from build123d import *

# Parameters (mm, degrees)
CHAMFER1_SIZE                   = 2
BOSS_EXTRUDE1_DEPTH             = 70
CHAMFER3_SIZE                   = 14
SKETCH7_R                       = 5
CUT_EXTRUDE1_DEPTH              = 70
CIRPATTERN4_COUNT               = 4
CHAMFER3_OF_CIRPATTERN4_SIZE    = 14
CUT_EXTRUDE3_START              = 70
CUT_EXTRUDE3_DEPTH              = 70
CUT_EXTRUDE4_DEPTH              = 70
CIRPATTERN5_COUNT               = 2
CIRPATTERN5_ANGLE               = 10
CIRPATTERN5_THE_OTHER_WAY_COUNT = 2
CIRPATTERN5_THE_OTHER_WAY_ANGLE = 10
CIRPATTERN7_COUNT               = 4
CIRPATTERN7_COPY_1_DEPTH        = 70
CIRPATTERN7_COPY_2_DEPTH        = 70
CIRPATTERN7_COPY_3_DEPTH        = 70
CIRPATTERN7_COPY_4_DEPTH        = 70
CIRPATTERN7_COPY_5_DEPTH        = 70
CIRPATTERN7_COPY_6_DEPTH        = 70
CUT_SWEEP2_PROFILE_R            = 0.5
CUT_SWEEP9_PROFILE_R            = 0.5
CUT_EXTRUDE5_START              = -10
SKETCH109_R                     = 37.5
CUT_EXTRUDE5_DEPTH              = 10


with BuildPart() as part:
    # Sketch1 → Revolve1 (revolve)
    with BuildSketch(Plane.XY, mode=Mode.PRIVATE) as revolve1_sk:
        Polygon((0, 0), (-50, 0), (-50, 28), (-37.5, 28), (-37.5, 31), (-5, 31), (-5, 41), (0, 41), align=None)
    revolve(revolve1_sk.sketch.rotate(Axis((0, 0, 0), (0, 1, 0)), 270), axis=Axis((0, 0, 0), (0, 1, 0)))

    # Chamfer1
    chamfer1_edges = [part.edges().sort_by_distance(p)[0] for p in [
        (0, 31, 37.5),
        (0, 28, 50),
    ]]
    chamfer(chamfer1_edges, length=CHAMFER1_SIZE)

    # Sketch3 → Boss-Extrude1 (add)
    with BuildSketch(Plane.XY):
        Polygon((-12.5, 26), (-12.5, 0), (12.5, 0), (12.5, 26), (10.5, 26), (10.5, 2), (-10.5, 2), (-10.5, 26), align=None)
    boss_extrude1 = extrude(amount=BOSS_EXTRUDE1_DEPTH)

    # Chamfer3
    chamfer3_edges = [part.edges().sort_by_distance(p)[0] for p in [
        (11.5, 26, 70),
        (-11.5, 26, 70),
    ]]
    chamfer(chamfer3_edges, length=CHAMFER3_SIZE)

    # Sketch7 → Cut-Extrude1 (cut)
    with BuildSketch(Plane(origin=(0, 0, 0), x_dir=(1, 0, 0), z_dir=(0, 1, 0))):
        with Locations(Location((0, -60, 0), (0, 0, 90))):
            Circle(SKETCH7_R)
    cut_extrude1 = extrude(amount=CUT_EXTRUDE1_DEPTH, mode=Mode.SUBTRACT)

    # CirPattern4: Boss-Extrude1, Cut-Extrude1 ×4 about axis
    cirpattern4_axis = Axis((0, 0, 0), (0, 1, 0))
    add([boss_extrude1.rotate(cirpattern4_axis, i * 360 / CIRPATTERN4_COUNT) for i in range(1, CIRPATTERN4_COUNT)])
    add([cut_extrude1.rotate(cirpattern4_axis, i * 360 / CIRPATTERN4_COUNT) for i in range(1, CIRPATTERN4_COUNT)], mode=Mode.SUBTRACT)

    # Chamfer3 of CirPattern4
    chamfer3_of_cirpattern4_edges = [part.edges().sort_by_distance(p)[0] for p in [
        (70, 26, -11.5),
        (70, 26, 11.5),
        (-11.5, 26, -70),
        (11.5, 26, -70),
        (-70, 26, 11.5),
        (-70, 26, -11.5),
    ]]
    chamfer(chamfer3_of_cirpattern4_edges, length=CHAMFER3_OF_CIRPATTERN4_SIZE)

    # Sketch12 → Cut-Extrude3 (cut)
    with BuildSketch(Plane(origin=(0, 0, 0), x_dir=(1, 0, 0), z_dir=(0, 1, 0)).offset(CUT_EXTRUDE3_START)):
        with BuildLine():
            Line((23.02513458, -42.117017672), (23.12024219, -44.333445626))
            ThreePointArc((23.12024219, -44.333445626), (35.355339059, -35.355339059), (44.333445626, -23.12024219))
            Line((44.333445626, -23.12024219), (42.117017672, -23.02513458))
            ThreePointArc((42.117017672, -23.02513458), (33.941125497, -33.941125497), (23.02513458, -42.117017672))
        make_face()
    cut_extrude3 = extrude(amount=-CUT_EXTRUDE3_DEPTH, mode=Mode.SUBTRACT)

    # Sketch19 → Cut-Extrude4 (cut)
    with BuildSketch(Plane(origin=(0, 0, 0), x_dir=(1, 0, 0), z_dir=(0, 1, 0))):
        Polygon((36.062317099, -33.941125497), (33.917754876, -36.038946478), (31.819933895, -33.894384255), (33.964496118, -31.796563274), align=None)
    cut_extrude4 = extrude(amount=CUT_EXTRUDE4_DEPTH, mode=Mode.SUBTRACT)

    # CirPattern5: Cut-Extrude4 ×2 about axis
    cirpattern5_axis = Axis((0, 0, 0), (0, -1, 0))
    for i in range(1, CIRPATTERN5_COUNT):
        add(cut_extrude4.rotate(cirpattern5_axis, i * CIRPATTERN5_ANGLE / (CIRPATTERN5_COUNT - 1)), mode=Mode.SUBTRACT)

    # CirPattern5 the other way: Cut-Extrude4 ×2 about axis
    cirpattern5_the_other_way_axis = Axis((0, 0, 0), (0, 1, 0))
    for i in range(1, CIRPATTERN5_THE_OTHER_WAY_COUNT):
        add(cut_extrude4.rotate(cirpattern5_the_other_way_axis, i * CIRPATTERN5_THE_OTHER_WAY_ANGLE / (CIRPATTERN5_THE_OTHER_WAY_COUNT - 1)), mode=Mode.SUBTRACT)

    # CirPattern7: Cut-Extrude3, Cut-Extrude4 ×4 about axis
    cirpattern7_axis = Axis((0, 0, 0), (0, 1, 0))
    add([cut_extrude3.rotate(cirpattern7_axis, i * 360 / CIRPATTERN7_COUNT) for i in range(1, CIRPATTERN7_COUNT)], mode=Mode.SUBTRACT)
    add([cut_extrude4.rotate(cirpattern7_axis, i * 360 / CIRPATTERN7_COUNT) for i in range(1, CIRPATTERN7_COUNT)], mode=Mode.SUBTRACT)

    # CirPattern7 copy 1 sketch → CirPattern7 copy 1 (cut)
    with BuildSketch(Plane(origin=(0, 0, 0), x_dir=(0.1736481776669308, 0, -0.984807753012208), z_dir=(0, 1, 0))):
        Polygon((36.062317099, -33.941125497), (33.917754876, -36.038946478), (31.819933895, -33.894384255), (33.964496118, -31.796563274), align=None)
    extrude(amount=CIRPATTERN7_COPY_1_DEPTH, mode=Mode.SUBTRACT)

    # CirPattern7 copy 2 sketch → CirPattern7 copy 2 (cut)
    with BuildSketch(Plane(origin=(0, 0, 0), x_dir=(-0.984807753012208, 0, -0.17364817766693086), z_dir=(0, 1, 0))):
        Polygon((36.062317099, -33.941125497), (33.917754876, -36.038946478), (31.819933895, -33.894384255), (33.964496118, -31.796563274), align=None)
    extrude(amount=CIRPATTERN7_COPY_2_DEPTH, mode=Mode.SUBTRACT)

    # CirPattern7 copy 3 sketch → CirPattern7 copy 3 (cut)
    with BuildSketch(Plane(origin=(0, 0, 0), x_dir=(-0.17364817766693094, 0, 0.984807753012208), z_dir=(0, 1, 0))):
        Polygon((36.062317099, -33.941125497), (33.917754876, -36.038946478), (31.819933895, -33.894384255), (33.964496118, -31.796563274), align=None)
    extrude(amount=CIRPATTERN7_COPY_3_DEPTH, mode=Mode.SUBTRACT)

    # CirPattern7 copy 4 sketch → CirPattern7 copy 4 (cut)
    with BuildSketch(Plane(origin=(0, 0, 0), x_dir=(-0.1736481776669307, 0, -0.984807753012208), z_dir=(0, 1, 0))):
        Polygon((36.062317099, -33.941125497), (33.917754876, -36.038946478), (31.819933895, -33.894384255), (33.964496118, -31.796563274), align=None)
    extrude(amount=CIRPATTERN7_COPY_4_DEPTH, mode=Mode.SUBTRACT)

    # CirPattern7 copy 5 sketch → CirPattern7 copy 5 (cut)
    with BuildSketch(Plane(origin=(0, 0, 0), x_dir=(-0.984807753012208, 0, 0.17364817766693064), z_dir=(0, 1, 0))):
        Polygon((36.062317099, -33.941125497), (33.917754876, -36.038946478), (31.819933895, -33.894384255), (33.964496118, -31.796563274), align=None)
    extrude(amount=CIRPATTERN7_COPY_5_DEPTH, mode=Mode.SUBTRACT)

    # CirPattern7 copy 6 sketch → CirPattern7 copy 6 (cut)
    with BuildSketch(Plane(origin=(0, 0, 0), x_dir=(0.17364817766693055, 0, 0.984807753012208), z_dir=(0, 1, 0))):
        Polygon((36.062317099, -33.941125497), (33.917754876, -36.038946478), (31.819933895, -33.894384255), (33.964496118, -31.796563274), align=None)
    extrude(amount=CIRPATTERN7_COPY_6_DEPTH, mode=Mode.SUBTRACT)

    # Cut-Sweep2: sweep along a path in Sketch27
    with BuildLine(Plane(origin=(0, 28, 0), x_dir=(1, 0, 0), z_dir=(0, 1, 0))) as cut_sweep2_path:
        CenterArc((0, 0), 41, 0, 360)
    # Cut-Sweep2 profile (on start of the path) → Cut-Sweep2 (sweep, cut)
    with BuildSketch(Plane(origin=(41, 28, 0), x_dir=(-1, 0, 0), z_dir=(0, 0, -1))):
        Circle(CUT_SWEEP2_PROFILE_R)
    sweep(path=cut_sweep2_path.line, mode=Mode.SUBTRACT)

    # Cut-Sweep9: sweep along a path in Sketch102
    with BuildLine(Plane(origin=(0, 28, 0), x_dir=(1, 0, 0), z_dir=(0, 1, 0))) as cut_sweep9_path:
        CenterArc((0, 0), 44, 0, 360)
    # Cut-Sweep9 profile (on start of the path) → Cut-Sweep9 (sweep, cut)
    with BuildSketch(Plane(origin=(44, 28, 0), x_dir=(-1, 0, 0), z_dir=(0, 0, -1))):
        Circle(CUT_SWEEP9_PROFILE_R)
    sweep(path=cut_sweep9_path.line, mode=Mode.SUBTRACT)

    # Sketch109 → Cut-Extrude5 (cut)
    with BuildSketch(Plane(origin=(0, 0, 0), x_dir=(-1, 0, 0), z_dir=(0, -1, 0)).offset(CUT_EXTRUDE5_START)):
        with Locations(Location((0, 0, 0), (0, 0, 90))):
            Circle(SKETCH109_R)
    extrude(amount=CUT_EXTRUDE5_DEPTH, mode=Mode.SUBTRACT)


solid = part.part
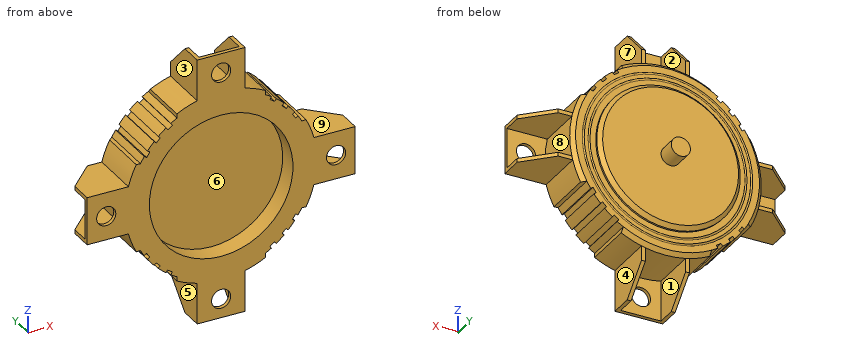
For this review, take the finished solid that the model builds, in its own axes (mm). Face numbers are marked on the shaded views. A direction names the side the tool comes from. Give positions to 0.01 mm unless a question says otherwise; leave off trailing zeros. Loops run counter-clockwise (first coordinate to the right, second up) from the corner with the lowest first, then second, coordinate; pieces in that order, holes last.
Item 1: Insertion check: pin 1 (23 mm diameter, centred on x = -3, z = -58.5, fed in from +Y); pin 2 (3 mm diameter, centred on x = 28.5, y = 7.5, fed in from -Z); pin 3 (17.5 mm diameter, centred on x = 62.5, y = 18, fed in from -Z); pin 4 (8 mm diameter, centred on x = -60, z = 0, fed in from -Y). Each pin has a flat end and moves straight along its axis. Give the tip position at first contact, or say it passes through.
Item 2: Draft analysis for pull direction Z (two halves, no side actions). For the marked faces 6, 7, 8 and 9, state which applies: +Z half, -Z half, draft (parallel to the pull), parting line (faces both ways), or undercut.
Item 3: Take a section at B-B, the plane z = -60. State the section outline as (x, y) points.
Item 4: Take a section at C-C, the plane z = 0. Give the number of separate pieces and of enclosed holes in the cut face, and give its area (3 significant figures).
Item 5: Tool access review of the marked faces 1, 2, 3, 4 and 5: name each direction out of +Z, -Z, +X, -X, +Y, -Y from which nothing blocks a thin tool from reaching the whole face with its end or side.
Item 6: For line 1 along X through (y, z) = (4.25, 0); line 2 along Z through (x, y) = (-60, 0.7), list the stretches that pass through material, from the lowest coordinate up.
Item 7: Take a section at D-D, the plane y = 37. State the section outline as (x, z) points.
Item 8: Take a section at A-A, the plane x = 60. State the section outline as (y, z) points.
Calculated:
1. pin 1: stops at y = 28
1. pin 2: stops at z = -38.45
1. pin 3: stops at z = -12.5
1. pin 4: passes through
2. face 6: undercut
2. face 7: draft
2. face 8: undercut
2. face 9: +Z half
3. outline: (-12.5, 0) - (-5, 0) - (-5, 2) - (-10.5, 2) - (-10.5, 22) - (-12.5, 22) - close; (5, 0) - (12.5, 0) - (12.5, 22) - (10.5, 22) - (10.5, 2) - (5, 2) - close
4. separate pieces: 3
4. enclosed holes: 0
4. area: 2,410 mm2
5. face 1: -Z, +Y
5. face 2: +Z, +Y
5. face 3: +Z, -X, +Y, -Y
5. face 4: -Z, +X, +Y, -Y
5. face 5: -Z, -X, +Y, -Y
6. line 1: x = -50 to -37.5, 37.5 to 50
6. line 2: z = -12.5 to -5, 5 to 12.5
7. outline: circle Ø10 at (0, 0)
8. outline: (0, -12.5) - (22, -12.5) - (22, -10.5) - (2, -10.5) - (2, -5) - (0, -5) - close; (0, 5) - (2, 5) - (2, 10.5) - (22, 10.5) - (22, 12.5) - (0, 12.5) - close
